CAD build for the part. Positions are in the model's coordinates, mm. A direction names the side the tool comes from. Coordinates: 2 decimals unless noted, no trailing zeros. Order: outer loops, then holes, each group sorted by start corner. A loop starts at its lowest first (then second) coordinate and runs counter-clockwise, first axis right, second up. Notation, with made-up numbers: M -16.5,52.25 L 9.5,52.25 A8 cw 9.5,64.25 Z; hole C -22,-30 d4. An arc over 180 degrees is marked long. Write item = value, one per line.
from build123d import *

# Parameters (mm, degrees)
F0_W     = 152.4
F0_H     = 101.6
F1_DEPTH = 76.2
F2_T     = -2.54
F3_R     = 1.25
F4_DEPTH = 2.541
F5_W     = 20.111805
F5_H     = 14.340593
F6_DEPTH = 25.4


with BuildPart() as f1:
    # F0 (on Top) → F1 (new body)
    with BuildSketch(Plane.XY):
        with Locations((15.56479, 5.227069)):
            Rectangle(F0_W, F0_H)
    extrude(amount=F1_DEPTH)

    # F2
    f2_openings = [f1.faces().sort_by_distance(p)[0] for p in [
        (15.56479, 5.227069, 76.2),
    ]]
    offset(amount=F2_T, openings=f2_openings)

    # F3 (on face) → F4 (cut, through all)
    with BuildSketch(Plane.XY.offset(2.54)):
        with Locations((21.336, -24.30905)):
            Circle(F3_R)
        with Locations((36.536, 26.49095)):
            Circle(F3_R)
        with Locations((64.436, 26.49095)):
            Circle(F3_R)
        with Locations((69.536, -24.30905)):
            Circle(F3_R)
    extrude(amount=-F4_DEPTH, mode=Mode.SUBTRACT)

    # F5 (on face) → F6 (cut)
    with BuildSketch(Plane.XZ.offset(45.572931)):
        with Locations((37.512888, 33.577968)):
            Rectangle(F5_W, F5_H)
    extrude(amount=-F6_DEPTH, mode=Mode.SUBTRACT)


solid = f1.part
(1) Wall check: line 1 (X direction, y = -5, z = 29); line 2 (Y direction, x = -47.5, z = 35); line 3 (Z direction, x = 62.5, y = 11.5). Give the ranges that are in metal, low to high. Write a range as from..to.
Evaluation:
line_1 = -60.64..-58.1, 89.22..91.76
line_2 = -45.57..-43.03, 53.49..56.03
line_3 = 0..2.54
(2) Pin check, flat tip, straight feed: pin 1 Ø3 at (x, y) = (19, 17) entering from +Z. Stop position of the tip, or through.
Evaluation:
pin_1 = 2.54
(3) Slice it at A-A, the plane z = 47. Write the cut outline in (x, y), then the cut area to 3 significant figures.
Evaluation:
outline = M -60.64,-45.57 L 91.76,-45.57 L 91.76,56.03 L -60.64,56.03 Z; hole M -58.1,-43.03 L 89.22,-43.03 L 89.22,53.49 L -58.1,53.49 Z
area = 1,260 mm²
(4) Slice it at B-B, the plane y = 47. Write the cut outline in (x, z).
Evaluation:
outline = M -60.64,0 L 91.76,0 L 91.76,76.2 L 89.22,76.2 L 89.22,2.54 L -58.1,2.54 L -58.1,76.2 L -60.64,76.2 Z
(5) Pull direction Y, two halves, no side cores. Call faces 1 (the face through (89.225, 5, 39)), 2 (the face through (14, -45.573, 38)), 3 (the face through (-60.635, 5, 38)): +Y half, -Y half, draft (parallel to the pull), parting line (faces both ways), or undercut.
Evaluation:
face_1 = undercut
face_2 = -Y half
face_3 = draft
(6) Slice it at C-C, the plane x = 72.5. Write the cut outline in (y, z), then the cut area to 3 significant figures.
Evaluation:
outline = M -45.57,0 L 56.03,0 L 56.03,76.2 L 53.49,76.2 L 53.49,2.54 L -43.03,2.54 L -43.03,76.2 L -45.57,76.2 Z
area = 632 mm²
(7) Tool access for faces 4 (the face through (-7.4, -43.5, 76.2)), 5 (the face through (15, 6, 2.54)): list every direction of +Z, -Z, +X, -X, +Y, -Y with a clear straight run to the whole face (end or side of a thin tool).
Evaluation:
face_4 = +Z, +X, -X, +Y, -Y
face_5 = +Z
